```python
from build123d import *

# Parameters (mm, degrees)
SKETCH1_R           = 12.5
BOSS_EXTRUDE1_DEPTH = 11
SKETCH2_R           = 11
BOSS_EXTRUDE2_DEPTH = 16.5
SKETCH3_R           = 9
BOSS_EXTRUDE3_DEPTH = 18.6
SKETCH4_R           = 5.75
BOSS_EXTRUDE4_DEPTH = 10.1
SKETCH5_R           = 11.75
CUT_EXTRUDE1_DEPTH  = 4.5
BOSS_EXTRUDE5_START = 2
SKETCH6_R           = 11.75
BOSS_EXTRUDE5_DEPTH = 2


# Read off the part's stored shape, not the designer's step: Dome1
with BuildPart() as part:
    # Sketch1 → Boss-Extrude1 (new body)
    with BuildSketch(Plane.XY):
        Circle(SKETCH1_R)
    extrude(amount=BOSS_EXTRUDE1_DEPTH)

    # Sketch2 → Boss-Extrude2 (add)
    with BuildSketch(Plane.XY.offset(11)):
        Circle(SKETCH2_R)
    extrude(amount=BOSS_EXTRUDE2_DEPTH)

    # Sketch3 → Boss-Extrude3 (add)
    with BuildSketch(Plane.XY.offset(27.5)):
        Circle(SKETCH3_R)
    extrude(amount=BOSS_EXTRUDE3_DEPTH)

    # Sketch4 → Boss-Extrude4 (add)
    with BuildSketch(Plane.XY.offset(46.1)):
        Circle(SKETCH4_R)
    extrude(amount=BOSS_EXTRUDE4_DEPTH)

    # Sketch5 → Cut-Extrude1 (cut)
    with BuildSketch(Plane(origin=(0, 0, 0), x_dir=(-1, 0, 0), z_dir=(0, 0, -1))):
        Circle(SKETCH5_R)
    extrude(amount=-CUT_EXTRUDE1_DEPTH, mode=Mode.SUBTRACT)

    # Sketch6 → Boss-Extrude5 (add)
    with BuildSketch(Plane(origin=(0, 0, 4.5), x_dir=(-1, 0, 0), z_dir=(0, 0, -1)).offset(BOSS_EXTRUDE5_START)):
        Circle(SKETCH6_R)
    extrude(amount=-BOSS_EXTRUDE5_DEPTH)

    # Dome1 outline → Dome1 (revolve)
    with BuildSketch(Plane.XZ):
        with BuildLine():
            Line((0, 2.500000012), (0, -3))
            ThreePointArc((0, -3), (6.48676538, -1.556953293), (11.75000001, 2.500000012))
            Line((11.75000001, 2.500000012), (0, 2.500000012))
        make_face()
    revolve(axis=Axis((0, 0, 0), (0, 0, 1)))


solid = part.part
```
Here's how the part is built. I have some questions about the finished solid (model axes, mm). A direction names the side the tool comes from. Coordinates: 2 decimals unless noted, no trailing zeros. Order: outer loops, then holes, each group sorted by start corner. A loop starts at its lowest first (then second) coordinate and runs counter-clockwise, first axis right, second up.
1) Imagine slicing it at A-A on x = 0. List the corners of the cut face in (y, z) for me, and give its area (3 significant figures).
2) I need wall thicknesses on line 1 (Y direction, x = 0, z = 1); line 2 (Y direction, x = 0, z = 1.35); line 3 (Z direction, x = 1.75, y = -0.75). Which ranges of each line are inside material? Lowest first, please.
3) Imagine slicing it at D-D on y = -8. List the corners of the cut face in (x, z) for me.
4) Will these pins go through, and if not, where does the flat tip stop? pin 1 (1.5 mm diameter, centred on x = 3, z = 32.5, fed in from +Y); pin 2 (12 mm diameter, centred on x = -6, z = 23.5, fed in from +Y); pin 3 (6 mm diameter, centred on x = -0.5, y = 9.5, fed in from -Z).
5) Imagine slicing it at C-C on z = 21. List the corners of the cut face in (x, y) for me, and give its area (3 significant figures).
6) Which directions (+Z, -Z, +X, -X, +Y, -Y) give clear straight access to the entire face, cutting with the end or side of a thin tool? Please do faces 1 (the face through (11, -5, 0)), 2 (the face through (11.923, 3.755, 5.423)), 3 (the face through (0, -6, 46.1)).
Response values:
1. outline: (-12.5, 0) - (-11.75, 0) - (-11.75, 2.5) arc R15.3 ccw to (11.75, 2.5) - (11.75, 0) - (12.5, 0) - (12.5, 11) - (11, 11) - (11, 27.5) - (9, 27.5) - (9, 46.1) - (5.75, 46.1) - (5.75, 56.2) - (-5.75, 56.2) - (-5.75, 46.1) - (-9, 46.1) - (-9, 27.5) - (-11, 27.5) - (-11, 11) - (-12.5, 11) - close
1. area: 1,120 mm2
2. line 1: y = -12.5 to -11.75, -10.32 to 10.32, 11.75 to 12.5
2. line 2: y = -12.5 to -11.75, -10.69 to 10.69, 11.75 to 12.5
2. line 3: z = -2.88 to 56.2
3. outline: (-9.6, 0) - (-8.61, 0) - (-8.61, 2.5) arc R13.04 ccw to (8.61, 2.5) - (8.61, 0) - (9.6, 0) - (9.6, 11) - (7.55, 11) - (7.55, 27.5) - (4.12, 27.5) - (4.12, 46.1) - (-4.12, 46.1) - (-4.12, 27.5) - (-7.55, 27.5) - (-7.55, 11) - (-9.6, 11) - close
4. pin 1: stops at y = 8.71
4. pin 2: stops at y = 11
4. pin 3: stops at z = -1.54
5. outline: circle Ø22 at (0, 0)
5. area: 380 mm2
6. face 1: -Z
6. face 2: +Z, -Z
6. face 3: +Z
